Autodesk Inventor part; units mm, degrees
ref_plane "YZ Plane" through (0, 0, 0) normal (1, 0, 0) x (0, 1, 0)
ref_plane "XZ Plane" through (0, 0, 0) normal (0, 1, 0) x (-1, 0, 0)
ref_plane "XY Plane" through (0, 0, 0) normal (0, 0, 1) x (1, 0, 0)
sketch "Sketch1" plane through (0, 0, 0) normal (0, 1, 0) x (-1, 0, 0)
  line L0 (-10.8, 8.5) -> (10.8, 8.5)
  line L1 (10.8, 8.5) -> (10.8, -8.5)
  line L2 (10.8, -8.5) -> (-10.8, -8.5)
  line L3 (-10.8, -8.5) -> (-10.8, 8.5)
  line L4 (-10.8, 8.5) -> (10.8, -8.5) construction
  line L5 (10.8, 8.5) -> (-10.8, -8.5) construction
  point P0 (0, 0)
  dimension "d0" = 21.6
  dimension "d1" = 17
extrude "Extrusion1" add sketch "Sketch1" along normal blind 2
sketch "Sketch2" plane through (0, 2, 0) normal (0, 1, 0) x (1, 0, 0)
  line L0 (-10.8, 8.5) -> (-10.8, -8.5)
  line L1 (-10.8, -8.5) -> (-7.8, -8.5)
  line L2 (-7.8, -8.5) -> (-7.8, 8.5)
  line L3 (-7.8, 8.5) -> (-10.8, 8.5)
  line L4 (-10.8, 8.5) -> (-10.8, -8.5)
  point P0 (0, 0)
  point P1 (-10.8, 0)
  point P2 (-10.8, 8.5)
  dimension "d4" = 3
  dimension "d5" = 17
extrude "Extrusion2" add sketch "Sketch2" along normal blind 12
sketch "Sketch3" plane through (-7.8, 2, 8.5) normal (1, 0, 0) x (0, 0, -1)
  circle A0 centre (8.5, 6) radius 3
  line L0 (0, 12) -> (17, 12)
  line L1 (17, 0) -> (17, 12)
  circle A1 centre (4.1699, 8.5) radius 1.2
  line L2 (0, -2) -> (0, 12)
  line L3 (0, 6) -> (17, 6) construction
  line L4 (1.8753, 9.8248) -> (15.1247, 2.1752) construction
  circle A2 centre (12.8301, 3.5) radius 1.2
  point P0 (8.5, -2)
  point P1 (8.5, 6)
  dimension "d8" = 6
  dimension "d9" = 6
  dimension "d10" = 8.5
  dimension "d11" = 2.4
  dimension "d12" = -30
  dimension "d13" = 5
  dimension "d14" = 2.4
  dimension "d15" = 5
extrude "Extrusion3" cut sketch "Sketch3" against normal blind 5
sketch "Sketch4" plane through (-10.8, 0, -8.5) normal (-1, 0, 0) x (0, 0, 1)
  circle A0 centre (8.5, 8) radius 3
  circle A1 centre (8.5, 8) radius 8.5
  line L0 (0, 0) -> (0, 14)
  circle A2 centre (8.5, 8) radius 12.6892
  line L1 (8.5, 8) -> (-4.1892, 8)
  line L2 (8.5, 8) -> (21.1892, 8)
  point P0 (8.5, 0)
  point P1 (17, 8)
  point P2 (0, 8)
  dimension "d18" = 17
extrude "Extrusion4" cut sketch "Sketch4" against normal blind 5 contours A1 L1 A2 L2 picked at (-2.5876, 9.6903)
sketch "Sketch5" plane through (-10.8, 0, -8.5) normal (-1, 0, 0) x (0, 0, 1)
  circle A0 centre (4.1699, 5.5) radius 1.2
  circle A1 centre (12.8301, 10.5) radius 1.2
  line L0 (4.1699, 5.5) -> (12.8301, 10.5) construction
  point P0 (8.5, 0)
  point P1 (8.5, 8)
extrude "Extrusion6" cut sketch "Sketch5" against normal blind 0.4
sketch "Sketch7" plane through (0, 0, 0) normal (0, -1, 0) x (1, 0, 0)
  line L0 (-10.8, -8.5) -> (-10.8, 8.5)
  line L1 (-10.8, 0.8) -> (10.8, 0.8)
  line L2 (10.8, 0.8) -> (10.8, -0.8)
  line L3 (10.8, -0.8) -> (-10.8, -0.8)
  line L4 (-10.8, -0.8) -> (-10.8, 0.8)
  line L5 (10.8, 8.5) -> (10.8, -8.5)
  point P0 (0, 0)
  dimension "d27" = 1.6
  dimension "d28" = 0.8
extrude "Extrusion7" add sketch "Sketch7" along normal blind 1
fillet "Fillet1" radius 2 2 edges at (10.8, 1, -8.5) (10.8, 1, 8.5)
sketch "Sketch9" plane through (-7.8, 2, 8.5) normal (1, 0, 0) x (0, 0, -1)
  line L0 (17, 0) -> (16, 0)
  line L1 (16, 0) -> (16, 4)
  line L2 (16, 4) -> (17, 4)
  line L3 (17, 4) -> (17, 0)
  point P0 (8.5, -2)
  dimension "d36" = 1
  dimension "d37" = 4
extrude "Extrusion9" add sketch "Sketch9" along normal blind 4
chamfer "Chamfer2" distance 4 angle 45 1 edges at (-3.8, 6, -8)
mirror "Mirror2" about plane through (0, 0, 0) normal (0, 0, 1) of "Extrusion9", "Chamfer2"
properties part number "Trzymak2"
Could you check a few things on this model? Use its own coordinates, in mm. A direction names the side the tool comes from. Round coordinates to 2 decimals unless told otherwise and drop trailing zeros. Loops run counter-clockwise (first coordinate to the right, second up) from the corner with the lowest first, then second, coordinate; pieces in that order, holes last. Notation, with made-up numbers: (-38, 78.25) - (16, 78.25) arc R35 ccw to (16, 110.25) - close; hole circle Ø9 at (23, 60.5). An arc over 180 degrees is marked (long way). Write item = value, one per line.
1) Imagine slicing it at C-C (x = 0.5). Please give me the cut outline in (y, z), and give its area (3 significant figures).
Computed:
outline = (-1, -0.8) - (0, -0.8) - (0, -8.5) - (2, -8.5) - (2, 8.5) - (0, 8.5) - (0, 0.8) - (-1, 0.8) - close
area = 35.6 mm2
2) If we mould it in two halves opening along Z, with no side actions, what happens to faces 1 (the flat face through (-5.8, 4, 8)), 2 (the cylindrical face through (-9.28, 9.33, 4.59)), 3 (the flat face through (-5, 2, -8.5))? For each: pulls with the +Z half, pulls with the -Z half, needs draft (parallel to the pull), parting line crosses it, or undercut.
Computed:
face_1 = needs draft
face_2 = undercut
face_3 = pulls with the -Z half
3) Imagine slicing it at B-B (y = 5.5). Please give me the cut outline in (x, z), and give its area (3 significant figures).
Computed:
outline = (-10.8, -8.5) - (-7.3, -8.5) - (-7.3, -7.5) - (-7.8, -7.5) - (-7.8, -5.53) - (-10.8, -5.53) - close; (-10.8, -3.13) - (-7.8, -3.13) - (-7.8, -1.66) - (-10.8, -1.66) - close; (-10.8, 1.66) - (-7.8, 1.66) - (-7.8, 7.5) - (-7.3, 7.5) - (-7.3, 8.5) - (-10.8, 8.5) - close
area = 34.9 mm2
4) I'm going to push flat-ended pins straight in: P1, Ø5, axis at x = -1.5, z = -0.5, coming from the +Y side; P2, Ø1, axis at x = 5.5, z = 3.5, coming from the -Y side; P3, Ø2, axis at y = 9, z = 5.5, coming from the +X side. Where does each tip first touch, or does it pass through?
Computed:
P1 = 2
P2 = 0
P3 = -7.8
5) Imagine slicing it at A-A (z = 0). Please give me the cut outline in (x, y), and give its area (3 significant figures).
Computed:
outline = (-10.8, -1) - (10.8, -1) - (10.8, 2) - (-7.8, 2) - (-7.8, 5) - (-10.8, 5) - close; (-10.8, 11) - (-7.8, 11) - (-7.8, 14) - (-10.8, 14) - close
area = 82.8 mm2
6) Imagine slicing it at D-D (y = 10.5). Please give me the cut outline in (x, z), and give its area (3 significant figures).
Computed:
outline = (-10.8, -8.12) - (-7.8, -8.12) - (-7.8, -1.66) - (-10.8, -1.66) - close; (-10.8, 1.66) - (-7.8, 1.66) - (-7.8, 3.13) - (-10.8, 3.13) - close; (-10.8, 5.53) - (-7.8, 5.53) - (-7.8, 8.12) - (-10.8, 8.12) - close
area = 31.6 mm2
7) I need wall thicknesses on line 1 along X through (y, z) = (10.5, -3.5); line 2 along Y through (x, z) = (-3.25, 3.25); line 3 along Y through (x, z) = (-8.5, 0). Which ranges of each line are inside material? Lowest first, please. Write a range as from..to.
Computed:
line_1 = -10.8..-7.8
line_2 = 0..2
line_3 = -1..5, 11..14
8) On a 3-axis mill with a long thin cutter (end or side, diameter ignored), from which of +Z, -Z, +X, -X, +Y, -Y can I reach the whole of each face in a straight line? I mean faces 4 (the flat face through (-0.2, -0.5, 0.8)), 5 (the flat face through (0.2, -0.5, -0.8)), 6 (the cylindrical face through (-9.321, 11.203, 7.873)), 7 (the flat face through (-6.3, 3.6, 7.5)). Say none if no direction works.
Computed:
face_4 = +Z, +X, -X, -Y
face_5 = -Z, +X, -X, -Y
face_6 = +Z, +X, -X, +Y
face_7 = +X, +Y
